Could you check a few things on this drawing? It's one solid part, dimensions in mm from its lowest x, y, z. Coordinates: 2 decimals unless noted, no trailing zeros. Loops run counter-clockwise (first coordinate to the right, second up) from the corner with the lowest first, then second, coordinate; pieces in that order, holes last. Notation, with made-up numbers: (19, 51.5) -> (49, 51.5) arc R3 ccw to (49, 55.5) -> close; hole circle Ø8 at (39, 31). An arc over 180 degrees is marked (long way). One line per question, with ' | ' between items. Start each with the question number.
(1) Suppose I cut it at B-B (x = 7.5). Please give me the cut outline in (y, z).
(2) If I drill on line 1 along Y through (x, z) = (29.5, 1.25); line 2 along X through (y, z) = (1, 4.75); line 3 along X through (y, z) = (1.5, 3), over which ranges is the centre line in solid material (lowest first)?
(3) Suppose I cut it at A-A (z = 4.5). Please give me the cut outline in (x, y).
(4) Suppose I cut it at C-C (x = 42.5). Please give me the cut outline in (y, z), plus the area to 3 significant figures.
(5) I'm going to push a flat-ended pin straight in: pin 1 Ø2.5 at (x, z) = (57.5, 4) entering from -Y. Where does the tip first touch, or does it pass through?
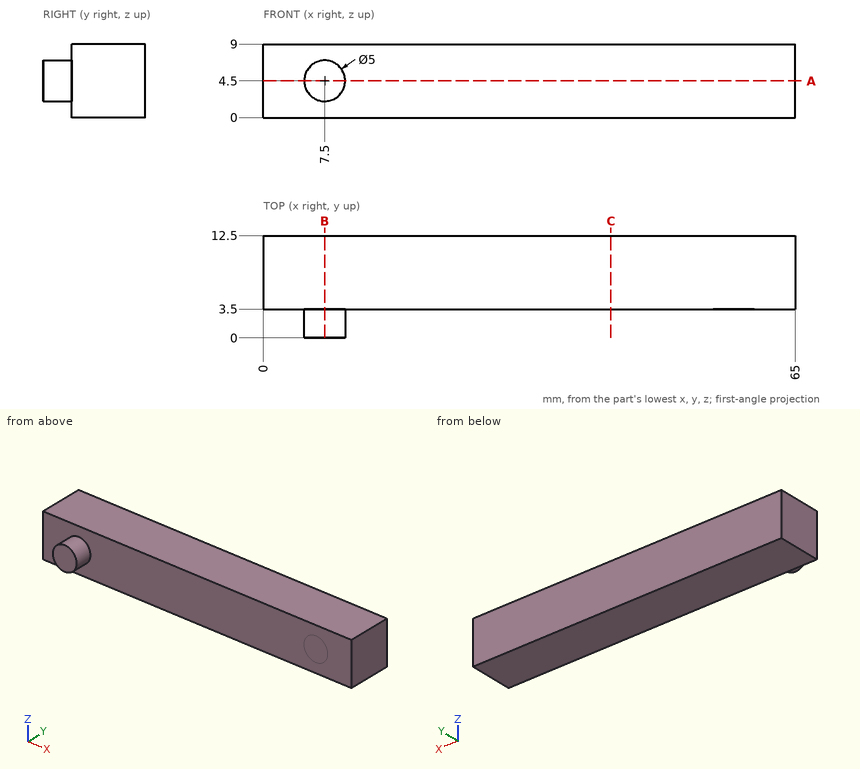
Checks:
1) outline: (0, 2) -> (3.5, 2) -> (3.5, 0) -> (12.5, 0) -> (12.5, 9) -> (3.5, 9) -> (3.5, 7) -> (0, 7) -> close
2) line 1: y = 3.5 to 12.5 | line 2: x = 5.01 to 9.99 | line 3: x = 5.5 to 9.5
3) outline: (0, 3.5) -> (5, 3.5) -> (5, 0) -> (10, 0) -> (10, 3.5) -> (65, 3.5) -> (65, 12.5) -> (0, 12.5) -> close
4) outline: (3.5, 0) -> (12.5, 0) -> (12.5, 9) -> (3.5, 9) -> close | area: 81.0 mm^2
5) pin 1: stops at y = 3.5
